Check sheet for the drawn part. Datum: minimum x, y, z corner. Units: mm. A direction names the side the tool comes from. Coordinates: 2 decimals unless noted, no trailing zeros. Write each loop counter-clockwise with the first axis right and the second up, starting at its lowest first coordinate (ties: lowest second). Pieces come first, ordered by that corner, then holes. Notation, with made-up numbers: M 4,56 L 63,56 A21 cw 63,95 Z; hole C 47.5,-1 d2. An arc over 180 degrees is marked long. Answer as a JSON object with one key per item and string values. Group by question number.
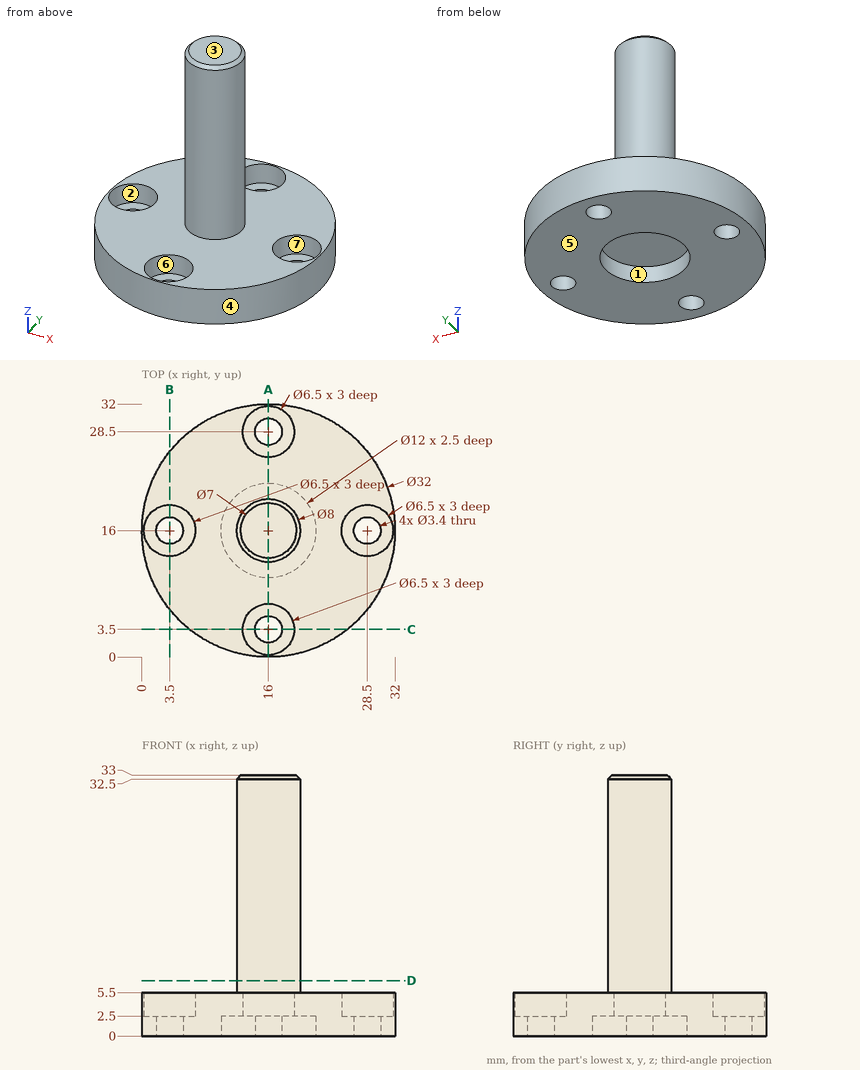
1) Go/stop test with flat-tipped pins: pin 1 Ø1 at (x, z) = (14, 5) entering from -Y; pin 2 Ø5 at (x, y) = (14.5, 8.5) entering from +Z; pin 3 Ø5 at (x, y) = (15.5, 28.5) entering from +Z. Record where each tip stops, or that it passes through.
2) Set-up check for the marked faces 1, 2 and 3: record each of +Z, -Z, +X, -X, +Y, -Y from which the full face is reachable in a straight line by a thin tool's end or side.
3) Section check D-D (z = 7). Record the cut outline in (x, y).
4) Section check A-A (x = 16). State how many separate pieces and enclosed holes the cut face has, then the cut area to 3 significant figures.
5) Section check B-B (x = 3.5). Record the cut outline in (y, z).
6) Draft check along X on the marked faces 4, 5, 6 and 7. Enter one of: +X half, -X half, draft (parallel to the pull), parting line (faces both ways), or undercut.
7) Material ranges on probe 1 along X at (y, z) = (16, 3.6); probe 2 along Z at (x, y) = (19, 2); probe 3 along Z at (x, y) = (14.5, 14.5), recorded low to high. Write a range as [from, to].
Entries:
{
 "1": {"pin 1": "y = 0.07", "pin 2": "z = 5.5", "pin 3": "z = 2.5"},
 "2": {"face 1": "-Z", "face 2": "+Z", "face 3": "+Z, +X, -X, +Y, -Y"},
 "3": {"outline": "C 16,16 d8"},
 "4": {"separate pieces": "3", "enclosed holes": "0", "area": "310 mm^2"},
 "5": {"outline": "M 6.01,0 L 14.3,0 L 14.3,2.5 L 12.75,2.5 L 12.75,5.5 L 6.01,5.5 Z; M 17.7,0 L 25.99,0 L 25.99,5.5 L 19.25,5.5 L 19.25,2.5 L 17.7,2.5 Z"},
 "6": {"face 4": "parting line", "face 5": "draft", "face 6": "undercut", "face 7": "undercut"},
 "7": {"probe 1": "[0, 0.25], [6.75, 25.25], [31.75, 32]", "probe 2": "[0, 5.5]", "probe 3": "[2.5, 33]"}
}
